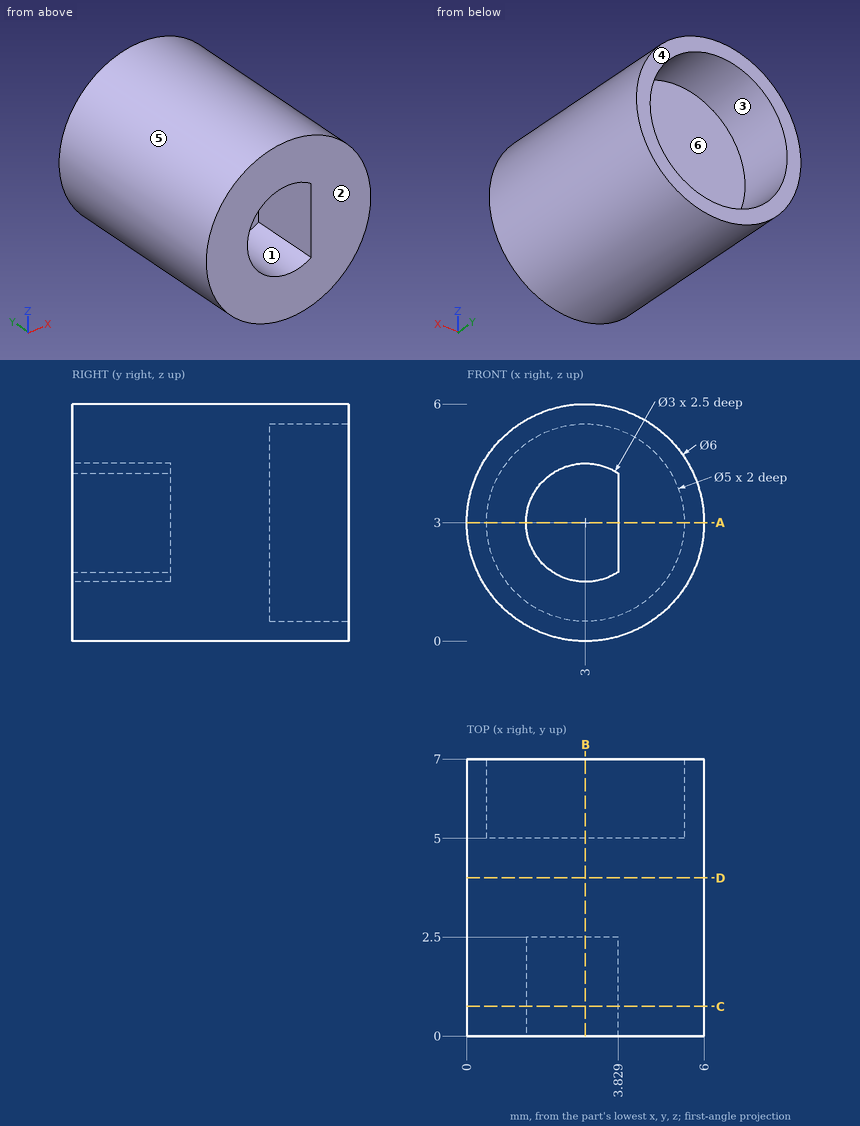
Print and shaded views of the part. All mm, measured from the part's lowest x, y and z. A direction names the side the tool comes from. Round coordinates to 2 decimals unless told otherwise and drop trailing zeros. Loops run counter-clockwise (first coordinate to the right, second up) from the corner with the lowest first, then second, coordinate; pieces in that order, holes last. Notation, with made-up numbers: (-38, 81) -> (-14, 81) arc R14 ccw to (-14, 104) -> close; hole circle Ø4 at (58.25, 66). An arc over 180 degrees is marked (long way). Use CSV: the item, a comma, the result in double quotes. Start each with the question number.
1) Pull direction Z, two halves, no side cores. Call the marked faces 4, 5 and 6: +Z half, -Z half, draft (parallel to the pull), parting line (faces both ways), or undercut.
2) Cut at D-D, the plane y = 4. Write the cut outline in (x, z), plus the area to 3 significant figures.
3) Drop flat-ended pins along their axis: P1, Ø1.5, axis at y = 4.5, z = 0.5, coming from the -X side; P2, Ø2.5, axis at x = 3, z = 3, coming from the +Y side. Give the stop position or say it passes through.
4) Cut at C-C, the plane y = 0.75. Write the cut outline in (x, z), plus the area to 3 significant figures.
5) Cut at A-A, the plane z = 3. Write the cut outline in (x, y).
6) Which spindle directions (+Z, -Z, +X, -X, +Y, -Y) get a long thin tool onto all of the face, cutting with end or side? Do the marked faces 1, 2 and 3. Say none if no direction does.
7) Wall check: L1, parallel to Z at x = 3, y = 5.55; L2, parallel to X at y = 1.5, z = 3.05; L3, parallel to Z at x = 3, y = 1.35. Give the ranges that are in metal, low to high. Write a range as [from, to].
8) Cut at B-B, the plane x = 3. Write the cut outline in (y, z).
Determined:
1,face 4,"draft"
1,face 5,"parting line"
1,face 6,"undercut"
2,outline,"circle Ø6 at (3, 3)"
2,area,"28.3 mm2"
3,P1,"stops at x = 0.56"
3,P2,"stops at y = 5"
4,outline,"circle Ø6 at (3, 3); hole (3.83, 1.75) -> (3.83, 4.25) arc R1.5 ccw (long way) to start"
4,area,"22.4 mm2"
5,outline,"(0, 0) -> (1.5, 0) -> (1.5, 2.5) -> (3.83, 2.5) -> (3.83, 0) -> (6, 0) -> (6, 7) -> (5.5, 7) -> (5.5, 5) -> (0.5, 5) -> (0.5, 7) -> (0, 7) -> close"
6,face 1,"-Y"
6,face 2,"+Z, -Z, +X, -X, -Y"
6,face 3,"+Y"
7,L1,"z = [0, 0.5], [5.5, 6]"
7,L2,"x = [0, 1.5], [3.83, 6]"
7,L3,"z = [0, 1.5], [4.5, 6]"
8,outline,"(0, 0) -> (7, 0) -> (7, 0.5) -> (5, 0.5) -> (5, 5.5) -> (7, 5.5) -> (7, 6) -> (0, 6) -> (0, 4.5) -> (2.5, 4.5) -> (2.5, 1.5) -> (0, 1.5) -> close"
